```python
from build123d import *

# Parameters (mm, degrees)
SKETCH001_R  = 65
PAD_DEPTH    = 4
SKETCH002_R  = 9.5
PAD001_DEPTH = 10


with BuildPart() as body001:
    # Sketch001 → Pad (new body)
    with BuildSketch(Plane.XY):
        Circle(SKETCH001_R)
    extrude(amount=PAD_DEPTH)


with BuildPart() as body002:
    # Sketch002 → Pad001 (new body)
    with BuildSketch(Plane.XY):
        Circle(SKETCH002_R)
    extrude(amount=PAD001_DEPTH)


with BuildPart() as body:
    # Sketch → Revolution (revolve)
    with BuildSketch(Plane.XZ):
        Polygon((4.5, 10), (4.5, 0), (56.757359, 0), (58.757359, 2), (61.242641, 2), (63.242641, 0), (95.232233, 0), (97, 1.767767), (97, 12.5), (96, 12.5), (96, 2.181981), (94.818019, 1), (63.656854, 1), (62.242641, 2.414214), (62.242641, 12.5), (61.242641, 12.5), (61.242641, 4), (57.928932, 4), (55.928932, 2), (9.5, 2), (9.5, 10), align=None)
    revolve(axis=Axis((0, 0, 0), (0, 0, 1)))

    # Boolean: intersect Body001
    add(body001.part, mode=Mode.INTERSECT)

    # Boolean001: intersect Body002
    add(body002.part, mode=Mode.INTERSECT)


solid = body.part
```
CAD build for the part. Positions are in the model's coordinates, mm. Give positions to 0.01 mm unless a question says otherwise; leave off trailing zeros. Loops run counter-clockwise (first coordinate to the right, second up) from the corner with the lowest first, then second, coordinate; pieces in that order, holes last. Notation, with made-up numbers: (48, -27.75) - (97, -27.75) arc R33 cw to (97, 4.25) - close; hole circle Ø11 at (3, 16). An arc over 180 degrees is marked (long way). Put each result on its own line as item: value.
Q1. Probe line 1 along Y through (x, z) = (0, 1.95); line 2 along X through (y, z) = (0.5, 3.3); line 3 along Y through (x, z) = (-1.25, 0.85). List the from-to ranges inside material, lowest first.
Filled in:
line 1: y = -9.5 to -4.5, 4.5 to 9.5
line 2: x = -9.49 to -4.47, 4.47 to 9.49
line 3: y = -9.42 to -4.32, 4.32 to 9.42
Q2. Slice it at D-D (x = -8). Give the cut face in (y, z).
Filled in:
outline: (-5.12, 0) - (5.12, 0) - (5.12, 4) - (-5.12, 4) - close
Q3. Slice it at A-A (x = 0). Give the cut face in (y, z).
Filled in:
outline: (-9.5, 0) - (-4.5, 0) - (-4.5, 4) - (-9.5, 4) - close; (4.5, 0) - (9.5, 0) - (9.5, 4) - (4.5, 4) - close
Q4. Flat gauge pins, fed straight in: pin 1 (1 mm diameter, centred on x = -2.5, z = 2.5, fed in from -Y); pin 2 (1.5 mm diameter, centred on y = 6, z = 2, fed in from -X). Where does each tip first touch, or does it go through?
Filled in:
pin 1: stops at y = -9.29
pin 2: stops at x = -7.92
Q5. Slice it at C-C (z = 3.1). Give the cut face in (x, y).
Filled in:
outline: circle Ø19 at (0, 0); hole circle Ø9 at (0, 0)
Q6. Mould opens along Y. For faces 1 (the face through (4.38, -8.43, 2.03)), 2 (the face through (-0.59, 4.46, 1.97)), 3 (the face through (-4.1, 2.2, 0)) say: pulls with the +Y half, pulls with the -Y half, needs draft (parallel to the pull), parting line crosses it, or undercut.
Filled in:
face 1: parting line crosses it
face 2: undercut
face 3: needs draft
